Can you work these out from the model? Positions are in its coordinate system, mm. Face numbers are marked on the shaded views. A direction names the side the tool comes from. Give positions to 0.01 mm unless a question says otherwise; leave off trailing zeros. Order: outer loops, then holes, each group sorted by start corner. A loop starts at its lowest first (then second) coordinate and runs counter-clockwise, first axis right, second up.
Item 1: I'm going to push flat-ended pins straight in: pin 1 Ø3 at (x, y) = (3, 5) entering from +Z; pin 2 Ø1 at (y, z) = (7.5, -5.5) entering from -X. Where does each tip first touch, or does it pass through?
Item 2: I want a section at C-C, the plane x = 0.75. Count the separate pieces of the cut face and the enclosed holes in it, then the cut area to 3 significant figures.
Item 3: If I drill on line 1 along Y through (x, z) = (4.5, 0); line 2 along Z through (x, y) = (5, -7.5); line 3 along Z through (x, y) = (4.75, -7), over which ranges is the centre line in solid material (lowest first)?
Item 4: I want a section at A-A, the plane y = 0. Write out the boundary of the cut face in (x, z), then the cut area to 3 significant figures.
Item 5: Which directions (+Z, -Z, +X, -X, +Y, -Y) give clear straight access to the entire face, cutting with the end or side of a thin tool? Please do the marked faces 4, 5, 6, 7 and 8.
Item 6: If we mould it in two halves opening along Y, with no side actions, what happens to the marked faces 1, 2 and 3? For each: +Y half, -Y half, draft (parallel to the pull), parting line (faces both ways), or undercut.
```python
from build123d import *

# Parameters (mm, degrees)
BASPROSKE_W             = 8
BASPROSKE_H             = 11
TOOTHCUT_DEPTH          = 18.492855685
TEETHCUTS_COUNT         = 20
TEETHCUTS_ANGLE         = 342
BORSKE_R                = 2
BORE_DEPTH              = 50.0000508
CUT_EXTRUDE1_DEPTH      = 6
CUT_EXTRUDE1_DEPTH_BACK = 13


with BuildPart() as part:
    # BasProSke → Base-Revolve (revolve)
    with BuildSketch(Plane(origin=(0, 0, 0), x_dir=(1, 0, 0), z_dir=(0, 1, 0)), mode=Mode.PRIVATE) as base_revolve_sk:
        with Locations((4, 5.5)):
            Rectangle(BASPROSKE_W, BASPROSKE_H)
    revolve(base_revolve_sk.sketch.rotate(Axis((-10, 0, 0), (1, 0, 0)), 180), axis=Axis((-10, 0, 0), (1, 0, 0)))

    # TooCutSke → ToothCut (cut, through all)
    with BuildSketch(Plane(origin=(0, 0, 0), x_dir=(0, 0, -1), z_dir=(1, 0, 0))):
        with BuildLine():
            ThreePointArc((0.499924007, 8.734705318), (0, 8.749), (-0.499924007, 8.734705318))
            ThreePointArc((-0.499924007, 8.734705318), (-0.824302243, 9.905497836), (-1.485192705, 10.924909509))
            ThreePointArc((-1.485192705, 10.924909509), (0, 11.0254), (1.485192705, 10.924909509))
            ThreePointArc((1.485192705, 10.924909509), (0.824302243, 9.905497836), (0.499924007, 8.734705318))
        make_face()
    toothcut = extrude(amount=TOOTHCUT_DEPTH, mode=Mode.SUBTRACT)

    # TeethCuts: ToothCut ×20 about axis
    teethcuts_axis = Axis((-10, 0, 0), (1, 0, 0))
    for i in range(1, TEETHCUTS_COUNT):
        add(toothcut.rotate(teethcuts_axis, i * TEETHCUTS_ANGLE / (TEETHCUTS_COUNT - 1)), mode=Mode.SUBTRACT)

    # BorSke → Bore (cut, symmetric)
    with BuildSketch(Plane(origin=(0, 0, 0), x_dir=(0, 0, -1), z_dir=(1, 0, 0))):
        with Locations(Location((0, 0, 0), (0, 0, 180))):
            Circle(BORSKE_R)
    extrude(amount=BORE_DEPTH, both=True, mode=Mode.SUBTRACT)

    # Sketch1 → Cut-Extrude1 (cut, two sides: drawn at the far end of the back side and taken through both)
    with BuildSketch(Plane(origin=(8, 0, 0), x_dir=(0, 0, -1), z_dir=(1, 0, 0)).offset(-CUT_EXTRUDE1_DEPTH_BACK)):
        with BuildLine():
            ThreePointArc((-2.5, -3.5), (-3.5, -2.5), (-4.5, -3.5))
            Line((-4.5, -3.5), (-2.5, -3.5))
        make_face()
        with BuildLine():
            Line((-2.5, -3.5), (-4.5, -3.5))
            ThreePointArc((-4.5, -3.5), (-4.207106781, -4.207106781), (-3.5, -4.5))
            ThreePointArc((-3.5, -4.5), (-2.792893219, -4.207106781), (-2.5, -3.5))
        make_face()
        with BuildLine():
            ThreePointArc((-3.499999992, 4.5), (-4.207106778, 4.207106784), (-4.5, 3.5))
            Line((-4.5, 3.5), (-2.5, 3.5))
            ThreePointArc((-2.5, 3.5), (-2.792893216, 4.207106778), (-3.499999992, 4.5))
        make_face()
        with BuildLine():
            Line((-2.5, 3.5), (-4.5, 3.5))
            ThreePointArc((-4.5, 3.5), (-4.207106779, 2.792893217), (-3.499999995, 2.5))
            ThreePointArc((-3.499999995, 2.5), (-2.792893217, 2.792893221), (-2.5, 3.5))
        make_face()
        with BuildLine():
            ThreePointArc((3.5, 2.5), (4.207106781, 2.792893219), (4.5, 3.5))
            Line((4.5, 3.5), (2.5, 3.5))
            ThreePointArc((2.5, 3.5), (2.792893219, 2.792893219), (3.5, 2.5))
        make_face()
        with BuildLine():
            Line((2.5, 3.5), (4.5, 3.5))
            ThreePointArc((4.5, 3.5), (4.207106781, 4.207106781), (3.5, 4.5))
            ThreePointArc((3.5, 4.5), (2.792893219, 4.207106781), (2.5, 3.5))
        make_face()
        with BuildLine():
            ThreePointArc((3.5, -4.5), (4.207106781, -4.207106781), (4.5, -3.5))
            Line((4.5, -3.5), (2.5, -3.5))
            ThreePointArc((2.5, -3.5), (2.792893219, -4.207106781), (3.5, -4.5))
        make_face()
        with BuildLine():
            Line((2.5, -3.5), (4.5, -3.5))
            ThreePointArc((4.5, -3.5), (4.207106781, -2.792893219), (3.5, -2.5))
            ThreePointArc((3.5, -2.5), (2.792893219, -2.792893219), (2.5, -3.5))
        make_face()
    extrude(amount=CUT_EXTRUDE1_DEPTH + CUT_EXTRUDE1_DEPTH_BACK, mode=Mode.SUBTRACT)


solid = part.part
```
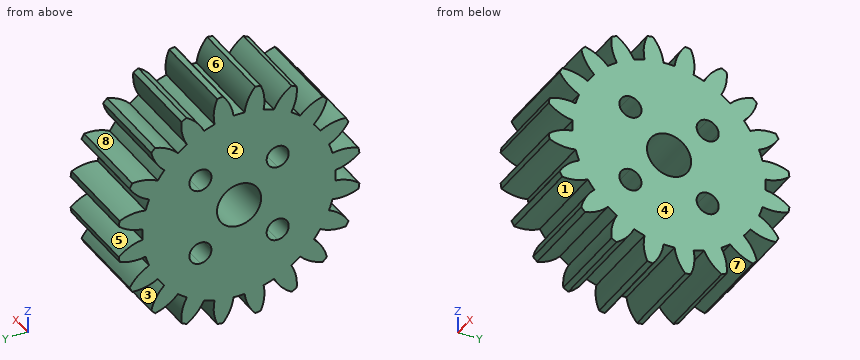
Results list:
1. pin 1: stops at z = 9.92
1. pin 2: passes through
2. separate pieces: 1
2. enclosed holes: 5
2. area: 278 mm2
3. line 1: y = -8.75 to -2, 2 to 8.75
3. line 2: z = -7.94 to -6.44, -4.8 to 4.8, 6.44 to 7.94
3. line 3: z = -7.78 to -5.77, -5.25 to 5.25, 5.77 to 7.78
4. outline: (0, -8.75) - (8, -8.75) - (8, -2) - (0, -2) - close; (0, 2) - (8, 2) - (8, 8.75) - (0, 8.75) - close
4. area: 108 mm2
5. face 4: +Z, -Z, +X, +Y, -Y
5. face 5: +X, -X, +Y
5. face 6: +Z, +X, -X
5. face 7: -Z, +X, -X
5. face 8: +X, -X
6. face 1: undercut
6. face 2: draft
6. face 3: +Y half
